from build123d import *

# Parameters (mm, degrees)
SKETCH1_W               = 40
SKETCH1_H               = 65.1
BOSS_EXTRUDE1_DEPTH     = 10
CUT_EXTRUDE1_DEPTH      = 10
SKETCH4_W               = 29.3
SKETCH4_H               = 59.5
CUT_EXTRUDE2_DEPTH      = 10
SKETCH5_R               = 1.5
CUT_EXTRUDE3_DEPTH      = 10
SKETCH7_W               = 10
SKETCH7_H               = 3
BOSS_EXTRUDE2_DEPTH     = 10
SKETCH8_W               = 10
SKETCH8_H               = 3
BOSS_EXTRUDE3_DEPTH     = 10
SKETCH9_R               = 1.65
CUT_EXTRUDE4_DEPTH      = 61
SKETCH10_R              = 1.65
CUT_EXTRUDE5_DEPTH      = 61
ESQUISSE1_W             = 15.35
ESQUISSE1_H             = 0.15
ESQUISSE1_W_2           = 29.3
ENL_V_MAT_EXTRU_1_DEPTH = 11


with BuildPart() as part:
    # Sketch1 → Boss-Extrude1 (new body)
    with BuildSketch(Plane.XY):
        with Locations((-0.1, 0)):
            Rectangle(SKETCH1_W, SKETCH1_H)
    extrude(amount=BOSS_EXTRUDE1_DEPTH)

    # Sketch2 → Cut-Extrude1 (cut)
    with BuildSketch(Plane.XY.offset(10)):
        Polygon((15, -32.55), (19.335, -27.45), (19.9, -27.45), (19.9, -32.55), align=None)
        Polygon((-20.1, -27.45), (-20.1, -32.55), (-15.2, -32.55), (-19.535, -27.45), align=None)
    extrude(amount=-CUT_EXTRUDE1_DEPTH, mode=Mode.SUBTRACT)

    # Sketch4 → Cut-Extrude2 (cut)
    with BuildSketch(Plane.XY.offset(10)):
        with Locations((-0.1, 2.8)):
            Rectangle(SKETCH4_W, SKETCH4_H)
    extrude(amount=-CUT_EXTRUDE2_DEPTH, mode=Mode.SUBTRACT)

    # Sketch5 → Cut-Extrude3 (cut)
    with BuildSketch(Plane.XY.offset(10)):
        with Locations((-17.4, 22.05)):
            Circle(SKETCH5_R)
        with Locations((-17.4, 0.05)):
            Circle(SKETCH5_R)
        with Locations((-17.4, -21.95)):
            Circle(SKETCH5_R)
        with Locations((-11.1, -29.75)):
            Circle(SKETCH5_R)
        with Locations((10.9, -29.75)):
            Circle(SKETCH5_R)
        with Locations((17.2, -21.95)):
            Circle(SKETCH5_R)
        with Locations((17.2, 0.05)):
            Circle(SKETCH5_R)
        with Locations((17.2, 22.05)):
            Circle(SKETCH5_R)
    extrude(amount=-CUT_EXTRUDE3_DEPTH, mode=Mode.SUBTRACT)

    # Sketch7 → Boss-Extrude2 (add)
    with BuildSketch(Plane(origin=(19.9, 0, 0), x_dir=(0, 0, -1), z_dir=(1, 0, 0))):
        with Locations((-5, 31.05)):
            Rectangle(SKETCH7_W, SKETCH7_H)
        with Locations((-5, -25.95)):
            Rectangle(SKETCH7_W, SKETCH7_H)
    extrude(amount=BOSS_EXTRUDE2_DEPTH)

    # Sketch8 → Boss-Extrude3 (add)
    with BuildSketch(Plane.ZY.offset(20.1)):
        with Locations((5, 31.05)):
            Rectangle(SKETCH8_W, SKETCH8_H)
        with Locations((5, -25.95)):
            Rectangle(SKETCH8_W, SKETCH8_H)
    extrude(amount=BOSS_EXTRUDE3_DEPTH)

    # Sketch9 → Cut-Extrude4 (cut, through all)
    with BuildSketch(Plane(origin=(0, -27.45, 0), x_dir=(-1, 0, 0), z_dir=(0, -1, 0))):
        with Locations((24.8175, -5)):
            Circle(SKETCH9_R)
    extrude(amount=-CUT_EXTRUDE4_DEPTH, mode=Mode.SUBTRACT)

    # Sketch10 → Cut-Extrude5 (cut, through all)
    with BuildSketch(Plane(origin=(0, -27.45, 0), x_dir=(-1, 0, 0), z_dir=(0, -1, 0))):
        with Locations((-24.6175, -5)):
            Circle(SKETCH10_R)
    extrude(amount=-CUT_EXTRUDE5_DEPTH, mode=Mode.SUBTRACT)

    # Esquisse1 → Enlèv. mat.-Extru.1 (cut, through all)
    with BuildSketch(Plane.XY.offset(10)):
        Polygon((29.9, -27.45), (29.9, -27.3), (19.335, -27.3), (19.185, -27.3), (19.185, -27.905597112), (27.185, -27.905597112), (27.185, -27.45), align=None)
        with Locations((22.225, 32.475)):
            Rectangle(ESQUISSE1_W, ESQUISSE1_H)
        Polygon((-27.385, -27.905597112), (-27.385, -27.45), (-30.1, -27.45), (-30.1, -27.3), (-19.535, -27.3), (-19.385, -27.3), (-19.385, -27.905597112), align=None)
        with Locations((-22.425, 32.475)):
            Rectangle(ESQUISSE1_W, ESQUISSE1_H)
        with Locations((-0.1, -27.025)):
            Rectangle(ESQUISSE1_W_2, ESQUISSE1_H)
    extrude(amount=-ENL_V_MAT_EXTRU_1_DEPTH, mode=Mode.SUBTRACT)


solid = part.part
The listing builds one solid part. Answer for the finished solid, in the listing's coordinates (mm). A direction names the side the tool comes from. Coordinates: 2 decimals unless noted, no trailing zeros. Order: outer loops, then holes, each group sorted by start corner. A loop starts at its lowest first (then second) coordinate and runs counter-clockwise, first axis right, second up.
Q1. Which of the six approach directions +Z, -Z, +X, -X, +Y, -Y give full straight-line access (tool end or side, diameter ignored) to faces 1 (the face through (27, -24.45, 5)), 2 (the face through (14.55, 2, 5)), 3 (the face through (-23, -27.3, 6))?
Q2. Given P1, Ø5, axis at x = -25, z = 4, coming from the +Y side; P2, Ø2.5, axis at x = -11.1, y = -29.75, coming from the -Z side; P3, Ø5, axis at y = 9, z = 6.5, coming from the -X side; P4, Ø6, axis at y = 24, z = 8.5, coming from the +X side, each flat-ended and moving along its own axis, determine where each tip first touches the part or whether it passes through.
Q3. A cutting plane is placed at A-A, the plane y = 4. Write down the section's boundary in (x, z), and give its area (3 significant figures).
Q4. A cutting plane is placed at B-B, the plane x = 10.9. Write down the section's boundary in (y, z), and give its area (3 significant figures).
Q5. For a pull along Y with two mould halves and no side action, classify faces 4 (the face through (0, -27.1, 5)), 5 (the face through (-27, 29.55, 5)), 6 (the face through (25.93, -25.89, 6)) as pulls with the +Y half, pulls with the -Y half, needs draft (parallel to the pull), parting line crosses it, or undercut.
Q6. A cutting plane is placed at C-C, the plane z = 1. State how many separate pieces and enclosed holes the cut face has, and give its area (3 significant figures).
Q7. Consider line 1 (X direction, y = -26.7, z = 5); line 2 (X direction, y = -16, z = 9.5); line 3 (Y direction, x = 23.5, z = 8.5). Determine where each line is inside the solid, lowest interval first.
Q8. A cutting plane is placed at D-D, the plane x = 17.2. Write down the section's boundary in (y, z), and give its area (3 significant figures).
Answers follow:
1. face 1: +Z, -Z, +X
1. face 2: +Z, -Z, +Y
1. face 3: +Z, -Z, -X, -Y
2. P1: stops at y = 32.4
2. P2: passes through
2. P3: stops at x = -20.1
2. P4: stops at x = 19.9
3. outline: (-20.1, 0) - (-14.75, 0) - (-14.75, 10) - (-20.1, 10) - close; (14.55, 0) - (19.9, 0) - (19.9, 10) - (14.55, 10) - close
3. area: 107 mm2
4. outline: (-32.55, 0) - (-31.25, 0) - (-31.25, 10) - (-32.55, 10) - close; (-28.25, 0) - (-27.1, 0) - (-27.1, 10) - (-28.25, 10) - close
4. area: 24.5 mm2
5. face 4: pulls with the +Y half
5. face 5: undercut
5. face 6: needs draft
6. separate pieces: 1
6. enclosed holes: 8
6. area: 884 mm2
7. line 1: x = -30.1 to -26.47, -23.17 to -14.75, 14.55 to 22.97, 26.27 to 29.9
7. line 2: x = -20.1 to -14.75, 14.55 to 19.9
7. line 3: y = -27.3 to -24.45, 29.55 to 32.4
8. outline: (-29.96, 0) - (-23.45, 0) - (-23.45, 10) - (-29.96, 10) - close; (-20.45, 0) - (-1.45, 0) - (-1.45, 10) - (-20.45, 10) - close; (1.55, 0) - (20.55, 0) - (20.55, 10) - (1.55, 10) - close; (23.55, 0) - (32.4, 0) - (32.4, 10) - (23.55, 10) - close
8. area: 534 mm2
